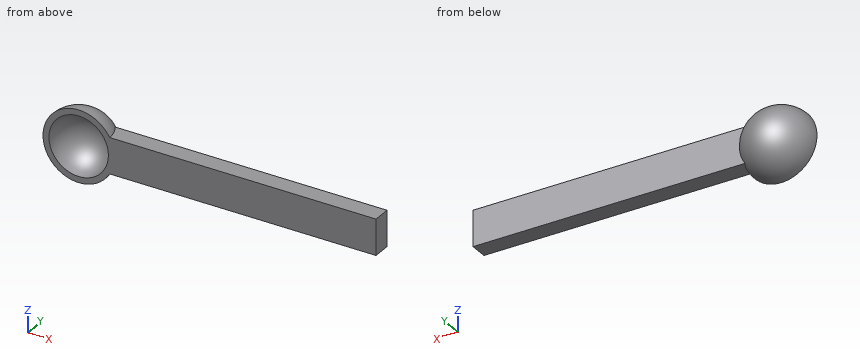
```python
from build123d import *

# Parameters (mm, degrees)
REVOLVE1_ANGLE                  = 180
BOSS_EXTRUDE1_REACH             = 20.111
BOSS_EXTRUDE1_END_RADIUS        = 6
SKETCH2_W                       = 6
SKETCH2_H                       = 3
BOSS_EXTRUDE1_DIRECTION_2_DEPTH = 40


with BuildPart() as part:
    # Sketch1 → Revolve1 (revolve)
    with BuildSketch(Plane(origin=(0, 0, 0), x_dir=(1, 0, 0), z_dir=(0, 1, 0))):
        with BuildLine():
            Line((-6, 0), (-5, 0))
            ThreePointArc((-5, 0), (0, 5), (5, 0))
            Line((5, 0), (6, 0))
            ThreePointArc((6, 0), (0, 6), (-6, 0))
        make_face()
    revolve(axis=Axis((-6, 0, 0), (1, 0, 0)), revolution_arc=REVOLVE1_ANGLE)

    # Boss-Extrude1: up to this sphere (the profile starts outside it)
    boss_extrude1_end = Location((0, 0, 0)) * Sphere(BOSS_EXTRUDE1_END_RADIUS, mode=Mode.PRIVATE)
    # Sketch2 → Boss-Extrude1 (add, up to the surface)
    with BuildSketch(Plane(origin=(10, 0, 0), x_dir=(0, 0, -1), z_dir=(1, 0, 0)), mode=Mode.PRIVATE) as boss_extrude1_sk1:
        with Locations((0, 1.5)):
            Rectangle(SKETCH2_W, SKETCH2_H)
    boss_extrude1_tool1 = extrude(boss_extrude1_sk1.sketch, amount=-BOSS_EXTRUDE1_REACH, mode=Mode.PRIVATE) - boss_extrude1_end
    add(boss_extrude1_tool1.solids().sort_by_distance((10, 1.5, 0))[0])

    # Sketch2 → Boss-Extrude1 direction 2 (add)
    with BuildSketch(Plane(origin=(10, 0, 0), x_dir=(0, 0, -1), z_dir=(1, 0, 0))):
        with Locations((0, 1.5)):
            Rectangle(SKETCH2_W, SKETCH2_H)
    extrude(amount=BOSS_EXTRUDE1_DIRECTION_2_DEPTH)


solid = part.part
```
For this review, take the finished solid that the model builds, in its own axes (mm). Coordinates: 2 decimals unless noted, no trailing zeros. Order: outer loops, then holes, each group sorted by start corner. A loop starts at its lowest first (then second) coordinate and runs counter-clockwise, first axis right, second up. Notation, with made-up numbers: (-38.75, 87) -> (18.25, 87) arc R26 cw to (18.25, 111) -> close; hole circle Ø6 at (58, -33). An arc over 180 degrees is marked (long way). Use CSV: the item, a comma, the result in double quotes. Start each with the question number.
Item 1: We need section A-A, the plane y = 1. Give the boundary of the cut face in (x, z), then the cut area to 3 significant figures.
Item 2: We need section C-C, the plane z = 2.5. Give the boundary of the cut face in (x, y), then the cut area to 3 significant figures.
Item 3: Insertion check: pin 1 (6 mm diameter, centred on x = 8, z = -4, fed in from +Y); pin 2 (0.9 mm diameter, centred on x = 26, y = 2, fed in from +Z); pin 3 (0.9 mm diameter, centred on x = 19, y = 2, fed in from -Z). Each pin has a flat end and moves straight along its axis. Give the tip position at first contact, or say it passes through.
Item 4: We need section D-D, the plane y = 4.25. Give the boundary of the cut face in (x, z).
Item 5: Wall thickness on probe 1 along Y at (x, z) = (25.5, -2.25); probe 2 along Z at (x, y) = (9, 0.75); probe 3 along X at (y, z) = (2, -1.75): over which ranges is each line inside the solid? List them lowest first.
Item 6: We need section B-B, the plane x = 7.5. Give the boundary of the cut face in (y, z).
Derived:
1,outline,"(5.1, -3) -> (50, -3) -> (50, 3) -> (5.1, 3) arc R5.92 ccw (long way) to start; hole circle Ø9.8 at (0, 0)"
1,area,"301 mm^2"
2,outline,"(-5.45, 0) -> (-4.33, 0) arc R4.33 cw to (4.33, 0) -> (50, 0) -> (50, 3) -> (4.56, 3) arc R5.45 ccw to start"
2,area,"152 mm^2"
3,pin 1,"stops at y = 3"
3,pin 2,"stops at z = 3"
3,pin 3,"stops at z = -3"
4,outline,"circle Ø8.47 at (0, 0); hole circle Ø5.27 at (0, 0)"
5,probe 1,"y = 0 to 3"
5,probe 2,"z = -3 to 3"
5,probe 3,"x = -5.38 to -4.24, 4.24 to 50"
6,outline,"(0, -3) -> (3, -3) -> (3, 3) -> (0, 3) -> close"
